Could you check a few things on this drawing? It's one solid part, dimensions in mm from its lowest x, y, z. A direction names the side the tool comes from. Give positions to 0.01 mm unless a question says otherwise; leave off trailing zeros. Order: outer loops, then holes, each group sorted by start corner. A loop starts at its lowest first (then second) coordinate and runs counter-clockwise, first axis right, second up.
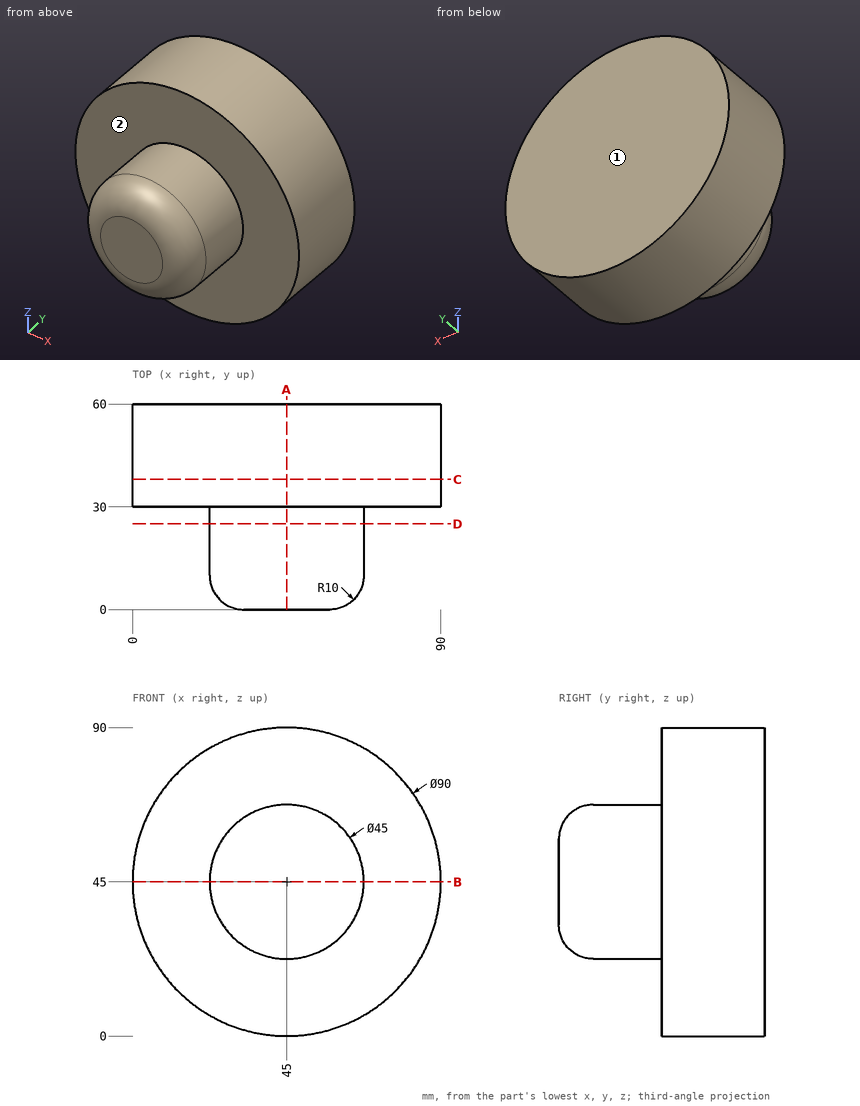
Q1. If we section it at B-B on z = 45: List the corners of the cut face in (x, y) for me.
Filled sheet:
outline: (0, 30) - (22.5, 30) - (22.5, 10) arc R10 ccw to (32.5, 0) - (57.5, 0) arc R10 ccw to (67.5, 10) - (67.5, 30) - (90, 30) - (90, 60) - (0, 60) - close
Q2. For the marked faces 1 and 2, which set-ups out of +Z, -Z, +X, -X, +Y, -Y let a thin tool reach every point of the face, with its end or its side?
Filled sheet:
face 1: +Z, -Z, +X, -X, +Y
face 2: -Y
Q3. I'm going to push flat-ended pins straight in: P1, Ø1, axis at x = 9.5, y = 37, coming from the +Z side; P2, Ø1.5, axis at x = 18.5, z = 60, coming from the -Y side; P3, Ø5, axis at x = 80.5, y = 53, coming from the -Z side. Where does each tip first touch, or does it pass through?
Filled sheet:
P1: stops at z = 73.28
P2: stops at y = 30
P3: stops at z = 14.41
Q4. I need wall thicknesses on L1, parallel to Y at x = 40, z = 75; L2, parallel to Z at x = 45, y = 49.5; L3, parallel to X at y = 11, z = 56. Which ranges of each line are inside material? Lowest first, please.
Filled sheet:
L1: y = 30 to 60
L2: z = 0 to 90
L3: x = 25.37 to 64.63
Q5. If we section it at A-A on x = 45: List the corners of the cut face in (y, z) for me, plus the area to 3 significant figures.
Filled sheet:
outline: (0, 32.5) arc R10 ccw to (10, 22.5) - (30, 22.5) - (30, 0) - (60, 0) - (60, 90) - (30, 90) - (30, 67.5) - (10, 67.5) arc R10 ccw to (0, 57.5) - close
area: 4,010 mm2
Q6. If we section it at C-C on y = 38: List the corners of the cut face in (x, z) for me, plus the area to 3 significant figures.
Filled sheet:
outline: circle Ø90 at (45, 45)
area: 6,360 mm2
Q7. If we section it at D-D on y = 25: List the corners of the cut face in (x, z) for me.
Filled sheet:
outline: circle Ø45 at (45, 45)
